Work out the finished part from the listing and answer in its coordinate system (mm). Give positions to 0.01 mm unless a question says otherwise; leave off trailing zeros. Order: outer loops, then holes, each group sorted by start corner. A loop starts at its lowest first (then second) coordinate and runs counter-clockwise, first axis right, second up.
```python
from build123d import *

# Parameters (mm, degrees)
SKETCH1_W                          = 50.8
SKETCH1_H                          = 6.35
BOSS_EXTRUDE1_DEPTH                = 2.032
F_1_16_0_0625_DIAMETER_HOLE1_D     = 1.5875
F_1_16_0_0625_DIAMETER_HOLE1_DEPTH = 70.104
F_1_16_0_0625_DIAMETER_HOLE1_TIP   = 0.476933116
F_1_8_0_125_DIAMETER_HOLE1_D       = 3.175
F_1_8_0_125_DIAMETER_HOLE1_DEPTH   = 70.104
F_1_8_0_125_DIAMETER_HOLE1_TIP     = 0.953866233


with BuildPart() as part:
    # Sketch1 → Boss-Extrude1 (new body)
    with BuildSketch(Plane(origin=(0, 0, 0), x_dir=(0, 0, -1), z_dir=(1, 0, 0))):
        with Locations((25.4, 3.175)):
            Rectangle(SKETCH1_W, SKETCH1_H)
    extrude(amount=BOSS_EXTRUDE1_DEPTH)

    # 1/16 (0.0625) Diameter Hole1
    with Locations(Plane(origin=(2.032, 0, 0), x_dir=(0, 0, -1), z_dir=(1, 0, 0))):
        with Locations((40.64, 3.175), (48.26, 3.175)):
            Hole(F_1_16_0_0625_DIAMETER_HOLE1_D / 2, depth=F_1_16_0_0625_DIAMETER_HOLE1_DEPTH)
            with Locations((0, 0, -(F_1_16_0_0625_DIAMETER_HOLE1_DEPTH + F_1_16_0_0625_DIAMETER_HOLE1_TIP / 2))):  # 118° drill point
                Cone(0, F_1_16_0_0625_DIAMETER_HOLE1_D / 2, F_1_16_0_0625_DIAMETER_HOLE1_TIP, mode=Mode.SUBTRACT)

    # 1/8 (0.125) Diameter Hole1
    with Locations(Plane(origin=(2.032, 0, 0), x_dir=(0, 0, -1), z_dir=(1, 0, 0))):
        with Locations((8.89, 3.175)):
            Hole(F_1_8_0_125_DIAMETER_HOLE1_D / 2, depth=F_1_8_0_125_DIAMETER_HOLE1_DEPTH)
            with Locations((0, 0, -(F_1_8_0_125_DIAMETER_HOLE1_DEPTH + F_1_8_0_125_DIAMETER_HOLE1_TIP / 2))):  # 118° drill point
                Cone(0, F_1_8_0_125_DIAMETER_HOLE1_D / 2, F_1_8_0_125_DIAMETER_HOLE1_TIP, mode=Mode.SUBTRACT)


solid = part.part
```
1. The part is cut by section A-A (z = -8.89). Write down the section's boundary in (x, y).
Findings below:
outline: (0, 0) - (2.03, 0) - (2.03, 1.59) - (0, 1.59) - close; (0, 4.76) - (2.03, 4.76) - (2.03, 6.35) - (0, 6.35) - close
2. Given P1, Ø1, axis at y = 3.175, z = -40.64, coming from the -X side; P2, Ø2.5, axis at y = 3.175, z = -48.26, coming from the +X side, each flat-ended and moving along its own axis, determine where each tip first touches the part or whether it passes through.
Findings below:
P1: passes through
P2: stops at x = 2.03
3. The part is cut by section B-B (x = 1.7). State how many separate pieces and enclosed holes the cut face has, then the cut area to 3 significant figures.
Findings below:
separate pieces: 1
enclosed holes: 3
area: 311 mm2
4. The mould has two halves that part along Y. Classify faces 1 (the face through (1, 4.75, -9.1)), 2 (the face through (1, 0, -25)), 3 (the face through (1.002, 3.21, -41.433)), 4 (the face through (1, 6.35, -25)): pulls with the +Y half, pulls with the -Y half, needs draft (parallel to the pull), parting line crosses it, or undercut.
Findings below:
face 1: undercut
face 2: pulls with the -Y half
face 3: undercut
face 4: pulls with the +Y half
5. The part is cut by section C-C (z = -40.64). Write down the section's boundary in (x, y), then the cut area to 3 significant figures.
Findings below:
outline: (0, 0) - (2.03, 0) - (2.03, 2.38) - (0, 2.38) - close; (0, 3.97) - (2.03, 3.97) - (2.03, 6.35) - (0, 6.35) - close
area: 9.68 mm2
6. Straight lines are drawn through the part: probe 1 along Z at (x, y) = (0.15, 2.5); probe 2 along Z at (x, y) = (1.2, 3); probe 3 along Y at (x, z) = (1.6, -8.89). For each, find the intervals that lie inside material, in ascending order.
Findings below:
probe 1: z = -50.8 to -48.68, -47.84 to -41.06, -40.22 to -10.33, -7.45 to 0
probe 2: z = -50.8 to -49.03, -47.49 to -41.41, -39.87 to -10.47, -7.31 to 0
probe 3: y = 0 to 1.59, 4.76 to 6.35
